```python
from build123d import *

# Parameters (mm, degrees)
SWEEP_THIN1_PROFILE_R   = 7.5
SWEEP_THIN1_PROFILE_R_2 = 6
SKETCH29_R              = 7.5
BOSS_EXTRUDE1_DEPTH     = 8
SKETCH30_R              = 6
BOSS_EXTRUDE2_DEPTH     = 8
SKETCH31_W              = 6
SKETCH31_H              = 6
CUT_EXTRUDE2_DEPTH      = 16


with BuildPart() as part:
    # Sweep-Thin1: sweep along a path in Sketch2
    with BuildLine(Plane.XY) as sweep_thin1_path:
        Line((0, 0), (-34.5, 0))
        ThreePointArc((-34.5, 0), (-45.106601718, 4.393398282), (-49.5, 15))
        Line((-49.5, 15), (-49.5, 110))
        ThreePointArc((-49.5, 110), (-45.106601718, 120.606601718), (-34.5, 125))
        Line((-34.5, 125), (-22, 125))
    # Sweep-Thin1 profile (on start of the path) → Sweep-Thin1 (sweep)
    with BuildSketch(Plane(origin=(0, 0, 0), x_dir=(0, -1, 0), z_dir=(-1, 0, 0))):
        Circle(SWEEP_THIN1_PROFILE_R)
        Circle(SWEEP_THIN1_PROFILE_R_2, mode=Mode.SUBTRACT)
    sweep(path=sweep_thin1_path.line)

    # Sketch27 → Revolve1 (revolve)
    with BuildSketch(Plane.XY, mode=Mode.PRIVATE) as revolve1_sk:
        with BuildLine():
            Line((-22, 132.5), (-22, 125))
            Line((-22, 125), (-19.5, 125))
            ThreePointArc((-19.5, 125), (-20.141458774, 128.952847075), (-22, 132.5))
        make_face()
    revolve(revolve1_sk.sketch.rotate(Axis((-22, 125, 0), (1, 0, 0)), 180), axis=Axis((-22, 125, 0), (1, 0, 0)))

    # Sketch29 → Boss-Extrude1 (add)
    with BuildSketch(Plane(origin=(0, 0, 0), x_dir=(0, 0, -1), z_dir=(1, 0, 0))):
        with Locations(Location((0, 0, 0), (0, 0, 270))):
            Circle(SKETCH29_R)
    extrude(amount=BOSS_EXTRUDE1_DEPTH)

    # Sketch30 → Boss-Extrude2 (add)
    with BuildSketch(Plane(origin=(8, 0, 0), x_dir=(0, 0, -1), z_dir=(1, 0, 0))):
        with Locations(Location((0, 0, 0), (0, 0, 90))):
            Circle(SKETCH30_R)
    extrude(amount=BOSS_EXTRUDE2_DEPTH)

    # Sketch31 → Cut-Extrude2 (cut)
    with BuildSketch(Plane(origin=(16, 0, 0), x_dir=(0, 0, -1), z_dir=(1, 0, 0))):
        Rectangle(SKETCH31_W, SKETCH31_H)
    extrude(amount=-CUT_EXTRUDE2_DEPTH, mode=Mode.SUBTRACT)


solid = part.part
```
Input: part model. Units: mm. Frame: model coordinates. A direction names the side the tool comes from. Coordinates: 2 decimals unless noted, no trailing zeros. Write each loop counter-clockwise with the first axis right and the second up, starting at its lowest first coordinate (ties: lowest second). Pieces come first, ordered by that corner, then holes.
1) Section A-A on x = -26.5. Output: boundary loops of the cut face in (y, z), and give its area (3 significant figures).
2) Set-up query: faces 1 (the cylindrical face through (-17, 6, 0)), 2 (the flat face through (8, 0, 3)), 3 (the flat face through (16, 0, -4)). Return all of +Z, -Z, +X, -X, +Y, -Y with unobstructed straight access to the full face (end or side cutting, diameter ignored); none if empty.
3) Section C-C on y = 47.5. Output: boundary loops of the cut face in (x, z).
4) Mould query, pull axis Y, two halves, no side actions, for faces 4 (the flat face through (8, 0, -3)), 5 (the cylindrical face through (11.944, 5.723, 1.802)), 6 (the flat face through (8, 3, 0)), 7 (the flat face through (8, -2, -6)). Classes: pulls with the +Y half, pulls with the -Y half, needs draft (parallel to the pull), parting line crosses it, or undercut.
5) Material intervals for line 1 along Z through (x, y) = (-28.25, 125); line 2 along Y through (x, z) = (-36.5, 2); line 3 along X through (y, z) = (83.5, -5.5), sorted ascending.
6) Pin query (flat end, axial travel): pin 1 Ø3 at (x, y) = (-38, 116) entering from -Z; pin 2 Ø6 at (x, z) = (-15.5, 4) entering from +Y; pin 3 Ø5 at (x, y) = (11.5, -0.5) entering from +Z. Return the tip coordinate at first contact, or that it passes through.
Check result:
1. outline: circle Ø15 at (0, 0); circle Ø15 at (125, 0); hole circle Ø12 at (0, 0); hole circle Ø12 at (125, 0)
1. area: 127 mm2
2. face 1: none
2. face 2: +X
2. face 3: +Z, -Z, +X, +Y, -Y
3. outline: circle Ø15 at (-49.5, 0); hole circle Ø12 at (-49.5, 0)
4. face 4: undercut
4. face 5: parting line crosses it
4. face 6: undercut
4. face 7: needs draft
5. line 1: z = -7.5 to -6, 6 to 7.5
5. line 2: y = -7.14 to -5.56, 5.87 to 7.49, 117.51 to 119.13, 130.56 to 132.14
5. line 3: x = -54.6 to -51.9, -47.1 to -44.4
6. pin 1: stops at z = -3.65
6. pin 2: stops at y = 7.43
6. pin 3: stops at z = 6
